The model under review builds one solid part; all positions refer to its coordinate system, in mm. A direction names the side the tool comes from. Coordinates: 2 decimals unless noted, no trailing zeros. Write each loop counter-clockwise with the first axis right and the second up, starting at its lowest first coordinate (ties: lowest second). Pieces come first, ordered by that corner, then holes. Notation, with made-up numbers: (88, 17) -> (142, 17) arc R18 ccw to (142, 31) -> close; hole circle Ø5 at (-19, -7.75). An arc over 180 degrees is marked (long way). Write each question's results on one line, items separated by ' | '.
```python
from build123d import *

# Parameters (mm, degrees)
F0_W     = 81.85713
F0_H     = 65.510846
F1_DEPTH = 51.816
F3_DEPTH = 78.994
F5_DEPTH = 42.672


with BuildPart() as f1:
    # F0 (on Top) → F1 (new body)
    with BuildSketch(Plane.XY):
        Rectangle(F0_W, F0_H)
    extrude(amount=F1_DEPTH)

    # F2 (on face) → F3 (cut)
    with BuildSketch(Plane.XY.offset(51.816)):
        with BuildLine():
            Line((40.928565, -23.338192), (40.928565, 23.338192))
            ThreePointArc((40.928565, 23.338192), (17.590373, 0), (40.928565, -23.338192))
        make_face()
    extrude(amount=-F3_DEPTH, mode=Mode.SUBTRACT)

    # F4 (on face) → F5 (cut)
    with BuildSketch(Plane(origin=(-40.928565, 0, 0), x_dir=(0, -1, 0), z_dir=(-1, 0, 0))):
        with BuildLine():
            Line((32.755423, 51.816), (0.557004, 51.816))
            ThreePointArc((0.557004, 51.816), (9.987702, 29.048279), (32.755423, 19.61758))
            Line((32.755423, 19.61758), (32.755423, 51.816))
        make_face()
        with BuildLine():
            ThreePointArc((32.755423, 19.61758), (55.523144, 29.048279), (64.953843, 51.816))
            ThreePointArc((64.953843, 51.816), (32.755423, 84.01442), (0.557004, 51.816))
            Line((0.557004, 51.816), (32.755423, 51.816))
            Line((32.755423, 51.816), (32.755423, 19.61758))
        make_face()
    extrude(amount=-F5_DEPTH, mode=Mode.SUBTRACT)


solid = f1.part
```
Q1. Clearance check with flat-ended pins moving along their axes: P1, Ø12, axis at y = 7, z = 16.5, coming from the +X side; P2, Ø1.5, axis at y = -17, z = 25, coming from the -X side; P3, Ø1, axis at y = -0.5, z = 36.5, coming from the +X side. State where each tip first meets the part, or that it passes through.
Solution:
P1: x = 21.55 | P2: x = 1.74 | P3: x = 17.61
Q2. Add section C-C (x = -25). Write out the cut boundary in (y, z).
Solution:
outline: (-32.76, 0) -> (32.76, 0) -> (32.76, 51.82) -> (-0.56, 51.82) arc R32.2 cw to (-32.76, 19.62) -> close
Q3. Draft analysis for pull direction Y (two halves, no side actions). For faces 1 (the cylindrical face through (-19.89, -9.74, 29.3)), 2 (the flat face through (40.929, 28, 26)), 3 (the cylindrical face through (17.596, 0.513, 26.271)), state which applies: pulls with the +Y half, pulls with the -Y half, needs draft (parallel to the pull), parting line crosses it, or undercut.
Solution:
face 1: pulls with the -Y half | face 2: needs draft | face 3: undercut
Q4. Add section D-D (y = -10.5). Write out the cut boundary in (x, z), plus the area to 3 significant figures.
Solution:
outline: (-40.93, 0) -> (20.09, 0) -> (20.09, 51.82) -> (1.74, 51.82) -> (1.74, 28.55) -> (-40.93, 28.55) -> close | area: 2,170 mm²
Q5. Add section B-B (z = 3). Write out the cut boundary in (x, y).
Solution:
outline: (-40.93, -32.76) -> (40.93, -32.76) -> (40.93, -23.34) arc R23.34 cw to (40.93, 23.34) -> (40.93, 32.76) -> (-40.93, 32.76) -> close
Q6. Machinability: for faces 4 (the flat face through (1.743, -20, 40)), 5 (the flat face through (40.929, -28, 26)), which of the approach directions +Z, -Z, +X, -X, +Y, -Y give a long, thin tool a straight path to every point of the face, cutting with its end or side? Answer none if there is none.
Solution:
face 4: +Z, -X, -Y | face 5: +Z, -Z, +X, +Y, -Y
Q7. For line 1 (Y direction, x = 30.5, z = 43.5); line 2 (Y direction, x = 22.5, z = 44.5); line 3 (X direction, y = -25, z = 28.5), list the stretches that pass through material, from the lowest coordinate up. Write a range as from..to.
Solution:
line 1: -32.76..-20.88, 20.88..32.76 | line 2: -32.76..-14.32, 14.32..32.76 | line 3: 1.74..40.93
Q8. Add section A-A (x = 30). Write out the cut boundary in (y, z), plus the area to 3 significant figures.
Solution:
outline: (-32.76, 0) -> (-20.62, 0) -> (-20.62, 51.82) -> (-32.76, 51.82) -> close; (20.62, 0) -> (32.76, 0) -> (32.76, 51.82) -> (20.62, 51.82) -> close | area: 1,260 mm²
